The drawing under review shows one solid part. Ordinate dimensions are in mm from its lowest x, y, z. A direction names the side the tool comes from. Coordinates: 2 decimals unless noted, no trailing zeros. Loops run counter-clockwise (first coordinate to the right, second up) from the corner with the lowest first, then second, coordinate; pieces in that order, holes last. Notation, with made-up numbers: M 20.25,-29 L 33.25,-29 A13 cw 33.25,-24 Z; hole C -31,16 d8. An arc over 180 degrees is marked long. Return JSON: item names as keys, results as strings.
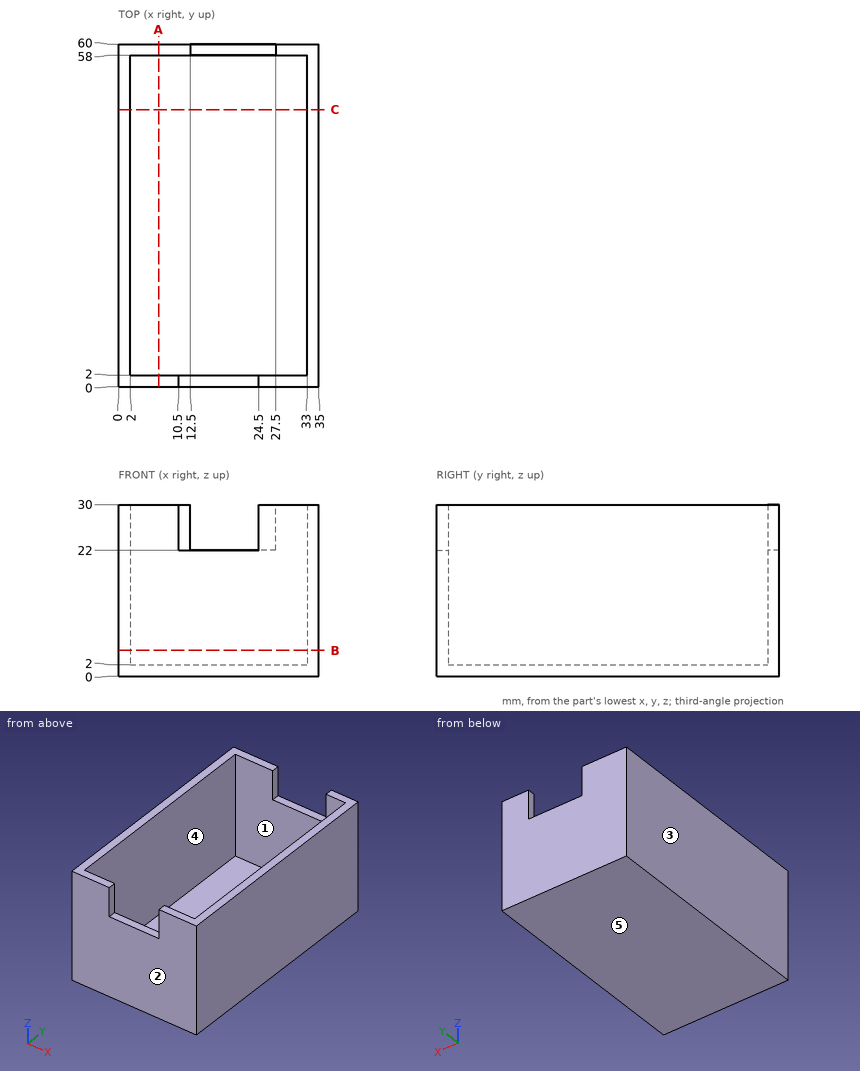
1. To check wall thickness, follow line 1 (Y direction, x = 32.5, z = 23); line 2 (X direction, y = 29, z = 17.75); line 3 (Z direction, x = 5.5, y = 5.5). State the ranges of each line that lie inside material, in increasing order.
Check values:
{"line 1": "0 to 2, 58 to 60", "line 2": "0 to 2, 33 to 35", "line 3": "0 to 2"}
2. The part is to be moulded in two halves that separate along Y. For the marked faces 1, 2 and 3, say which applies: released by +Y, released by -Y, zero draft, split by the parting line, or undercut.
Check values:
{"face 1": "undercut", "face 2": "released by -Y", "face 3": "zero draft"}
3. Add section C-C on y = 48.5. Give the boundary of the cut face in (x, z).
Check values:
{"outline": "M 0,0 L 35,0 L 35,30 L 33,30 L 33,2 L 2,2 L 2,30 L 0,30 Z"}
4. Add section A-A on x = 7. Give the boundary of the cut face in (y, z), plus the area to 3 significant figures.
Check values:
{"outline": "M 0,0 L 60,0 L 60,30 L 58,30 L 58,2 L 2,2 L 2,30 L 0,30 Z", "area": "232 mm²"}
5. Insertion check: pin 1 Ø9.5 at (x, y) = (24.5, 43.5) entering from +Z; pin 2 Ø2 at (x, y) = (16, 1.5) entering from +Z. Each pin has a flat end and moves straight along its axis. Give the tip position at first contact, or say it passes through.
Check values:
{"pin 1": "z = 2", "pin 2": "z = 22"}
6. Machinability: for the marked faces 4 and 5, which of the approach directions +Z, -Z, +X, -X, +Y, -Y give a long, thin tool a straight path to every point of the face, cutting with its end or side? Answer none if there is none.
Check values:
{"face 4": "+Z", "face 5": "-Z, +X, -X, +Y, -Y"}
7. Add section B-B on z = 4.5. Give the boundary of the cut face in (x, y), plus the area to 3 significant figures.
Check values:
{"outline": "M 0,0 L 35,0 L 35,60 L 0,60 Z; hole M 2,2 L 33,2 L 33,58 L 2,58 Z", "area": "364 mm²"}
